from build123d import *

# Parameters (mm, degrees)
F1_DEPTH = 10
F2_R     = 1


with BuildPart() as f1:
    # F0 (on Top) → F1 (new body)
    with BuildSketch(Plane.XY):
        with BuildLine():
            ThreePointArc((-41.8554165609, 24.0516047226), (-43.0993757866, 32.8488859903), (-35.2054165609, 28.7715093827))
            ThreePointArc((-35.2054165609, 28.7715093827), (-36.1280399533, 25.877550157), (-38.5554165609, 24.0516047226))
            Line((-38.5554165609, 24.0516047226), (-38.5554165609, 22.4844194358))
            ThreePointArc((-38.5554165609, 22.4844194358), (-37.7866546618, 22.738302037), (-37.0554165609, 23.0857816368))
            ThreePointArc((-37.0554165609, 23.0857816368), (-34.605193351, 25.4718881923), (-33.7054165609, 28.7715093827))
            ThreePointArc((-33.7054165609, 28.7715093827), (-43.5050377512, 34.3717325925), (-43.3554165609, 23.0857816368))
            ThreePointArc((-43.3554165609, 23.0857816368), (-42.6241784599, 22.738302037), (-41.8554165609, 22.4844194358))
            Line((-41.8554165609, 22.4844194358), (-41.8554165609, 24.0516047226))
        make_face()
        with BuildLine():
            ThreePointArc((-37.0554165609, 23.0857816368), (-37.7866546618, 22.738302037), (-38.5554165609, 22.4844194358))
            Line((-38.5554165609, 22.4844194358), (-38.5554165609, 19.9357816368))
            Line((-38.5554165609, 19.9357816368), (-37.0554165609, 19.9357816368))
            Line((-37.0554165609, 19.9357816368), (-37.0554165609, 21.4357816368))
            Line((-37.0554165609, 21.4357816368), (-37.0554165609, 23.0857816368))
        make_face()
        with BuildLine():
            Line((-41.8554165609, 19.9357816368), (-41.8554165609, 22.4844194358))
            ThreePointArc((-41.8554165609, 22.4844194358), (-42.6241784599, 22.738302037), (-43.3554165609, 23.0857816368))
            Line((-43.3554165609, 23.0857816368), (-43.3554165609, 21.4357816368))
            Line((-43.3554165609, 21.4357816368), (-43.3554165609, 19.9357816368))
            Line((-43.3554165609, 19.9357816368), (-41.8554165609, 19.9357816368))
        make_face()
        Polygon((-43.3554165609, 19.9357816368), (-43.3554165609, 21.4357816368), (-44.8554165609, 21.4357816368), align=None)
        Polygon((-35.5554165609, 21.4357816368), (-37.0554165609, 21.4357816368), (-37.0554165609, 19.9357816368), align=None)
    extrude(amount=F1_DEPTH)

    # F2
    f2_edges = [f1.edges().sort_by_distance(p)[0] for p in [
        (-43.355417, 19.935782, 5),
        (-37.055417, 19.935782, 5),
        (-41.855417, 19.935782, 5),
        (-41.855417, 24.051605, 5),
        (-37.055417, 23.085782, 5),
        (-43.355417, 23.085782, 5),
        (-38.555417, 24.051605, 5),
        (-38.555417, 19.935782, 5),
    ]]
    fillet(f2_edges, radius=F2_R)


solid = f1.part
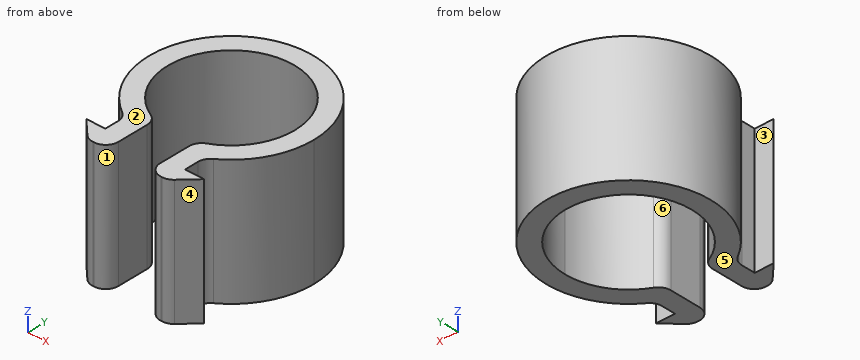
Input: part model. Units: mm. Frame: model coordinates. Face numbers are marked on the shaded views. A direction names the side the tool comes from. Coordinates: 2 decimals unless noted, no trailing zeros. Loops run counter-clockwise (first coordinate to the right, second up) from the corner with the lowest first, then second, coordinate; pieces in that order, holes last. Notation, with made-up numbers: (74, 1.25) -> (96, 1.25) arc R31 cw to (96, 33.25) -> close; hole circle Ø3 at (88.5, -13). An arc over 180 degrees is marked (long way). Write each question's results on one line, items separated by ' | '. Start each with the question number.
Q1. Section B-B, the plane x = -44.5. Return the cut outline in (y, z).
Q2. Pin query (flat end, axial travel): pin 1 (1.5 mm diameter, centred on y = 26, z = 2.5, fed in from +X); pin 2 (2 mm diameter, centred on y = 22.5, z = 3, fed in from -X); pin 3 (6 mm diameter, centred on x = -40.21, y = 28.77, fed in from -Z); pin 4 (1 mm diameter, centred on x = -44, z = 4, fed in from +Y). Return the tip coordinate at first contact, or that it passes through.
Q3. Reachability of the marked faces 1, 2 and 3 from +Z, -Z, +X, -X, +Y, -Y: full face, straight path, thin tool, end or side. Return the list, or none.
Q4. Pull-direction query (X, two-part tool) for the marked faces 4, 5 and 6; classes: released by +X, released by -X, zero draft, split by the parting line, or undercut.
Q5. Ray query, line 1 (Y direction, x = -36.75, z = 3.25); line 2 (X direction, y = 28.75, z = 3); line 3 (Y direction, x = -36, z = 3). Return the intervals inside material, ascending. Write a range as from..to.
Q6. Section C-C, the plane z = 6.5. Return the cut outline in (x, y).
Q7. Section D-D, the plane y = 25.5. Return the cut outline in (x, z), plus the area to 3 significant figures.
Q8. Section A-A, the plane y = 22.25. Return the cut outline in (x, z).
Found:
1) outline: (21.08, 0) -> (21.44, 0) -> (21.44, 10) -> (21.08, 10) -> close; (23.89, 0) -> (26.21, 0) -> (26.21, 10) -> (23.89, 10) -> close; (31.33, 0) -> (33.65, 0) -> (33.65, 10) -> (31.33, 10) -> close
2) pin 1: x = -34.03 | pin 2: x = -44.01 | pin 3: through | pin 4: y = 34.37
3) face 1: +Z, -Z, -Y | face 2: +Z, +X, -X, +Y, -Y | face 3: +Z, -Z, -X
4) face 4: released by +X | face 5: zero draft | face 6: undercut
5) line 1: 20.24..21.44, 23.24..25.16, 32.39..34.28 | line 2: -46.71..-45.21, -35.21..-33.71 | line 3: 20.99..21.44, 23.82..26.07, 31.48..33.73
6) outline: (-44.86, 21.44) -> (-43.65, 20.23) arc R1 ccw to (-42.94, 19.94) -> (-42.86, 19.94) arc R1 ccw to (-41.86, 20.94) -> (-41.86, 23.39) arc R1 ccw to (-42.41, 24.29) arc R5 cw (long way) to (-38, 24.29) arc R1 ccw to (-38.56, 23.39) -> (-38.56, 20.94) arc R1 ccw to (-37.56, 19.94) -> (-37.47, 19.94) arc R1 ccw to (-36.76, 20.23) -> (-35.56, 21.44) -> (-37.06, 21.44) -> (-37.06, 22.52) arc R1 cw to (-36.61, 23.36) arc R6.5 ccw (long way) to (-43.8, 23.36) arc R1 cw to (-43.36, 22.52) -> (-43.36, 21.44) -> close
7) outline: (-45.82, 0) -> (-43.99, 0) -> (-43.99, 10) -> (-45.82, 10) -> close; (-36.42, 0) -> (-34.59, 0) -> (-34.59, 10) -> (-36.42, 10) -> close | area: 36.7 mm2
8) outline: (-43.36, 0) -> (-41.86, 0) -> (-41.86, 10) -> (-43.36, 10) -> close; (-38.56, 0) -> (-37.06, 0) -> (-37.06, 10) -> (-38.56, 10) -> close
